from build123d import *

# Parameters (mm, degrees)
F0_W     = 550
F0_H     = 400
F1_DEPTH = 10
F2_W     = 9
F2_H     = 20
F2_H_2   = 70
F2_H_3   = 10
F2_H_4   = 75
F2_H_5   = 15
F2_H_6   = 18
F3_DEPTH = 5


with BuildPart() as f1:
    # F0 (on Front) → F1 (new body)
    with BuildSketch(Plane.XZ):
        Rectangle(F0_W, F0_H)
    extrude(amount=F1_DEPTH)

    # F2 (on face) → F3 (cut)
    with BuildSketch(Plane.XZ.offset(10)):
        Polygon((-218.013464, -37.5), (-215.013464, -37.5), (-215.013464, 37.5), (-218.013464, 37.5), (-227.013464, 37.5), (-230.013464, 37.5), (-230.013464, -37.5), (-227.013464, -37.5), align=None)
        with Locations((-222.513464, -47.5)):
            Rectangle(F2_W, F2_H)
        with Locations((-222.513464, 72.5)):
            Rectangle(F2_W, F2_H_2)
        Polygon((219.224181, -40.562903), (222.224181, -40.562903), (222.224181, 29.437097), (219.224181, 29.437097), (210.224181, 29.437097), (207.224181, 29.437097), (207.224181, -40.562903), (210.224181, -40.562903), align=None)
        with Locations((214.724181, -45.562903)):
            Rectangle(F2_W, F2_H_3)
        with Locations((214.724181, 66.937097)):
            Rectangle(F2_W, F2_H_4)
        Polygon((-172.425557, -35.359889), (-169.425557, -35.359889), (-169.425557, 29.640111), (-172.425557, 29.640111), (-181.425557, 29.640111), (-184.425557, 29.640111), (-184.425557, -35.359889), (-181.425557, -35.359889), align=None)
        with Locations((-176.925557, -40.359889)):
            Rectangle(F2_W, F2_H_3)
        with Locations((-176.925557, 67.140111)):
            Rectangle(F2_W, F2_H_4)
        Polygon((-124.808628, -20.359889), (-121.808628, -20.359889), (-121.808628, 59.640111), (-124.808628, 59.640111), (-133.808628, 59.640111), (-136.808628, 59.640111), (-136.808628, -20.359889), (-133.808628, -20.359889), align=None)
        with Locations((-129.308628, -27.859889)):
            Rectangle(F2_W, F2_H_5)
        with Locations((-129.308628, 69.640111)):
            Rectangle(F2_W, F2_H)
        Polygon((-73.533672, -28.500006), (-70.533672, -28.500006), (-70.533672, 36.499994), (-73.533672, 36.499994), (-82.533672, 36.499994), (-85.533672, 36.499994), (-85.533672, -28.500006), (-82.533672, -28.500006), align=None)
        with Locations((-78.033672, -33.500006)):
            Rectangle(F2_W, F2_H_3)
        with Locations((-78.033672, 41.499994)):
            Rectangle(F2_W, F2_H_3)
        Polygon((-19.896116, -21.071613), (-16.896116, -21.071613), (-16.896116, 38.928387), (-19.896116, 38.928387), (-28.896116, 38.928387), (-31.896116, 38.928387), (-31.896116, -21.071613), (-28.896116, -21.071613), align=None)
        with Locations((-24.396116, -28.571613)):
            Rectangle(F2_W, F2_H_5)
        with Locations((-24.396116, 43.928387)):
            Rectangle(F2_W, F2_H_3)
        Polygon((46.493838, -21.071613), (49.493838, -21.071613), (49.493838, 38.928387), (46.493838, 38.928387), (37.493838, 38.928387), (34.493838, 38.928387), (34.493838, -21.071613), (37.493838, -21.071613), align=None)
        with Locations((41.993838, -28.571613)):
            Rectangle(F2_W, F2_H_5)
        with Locations((41.993838, 43.928387)):
            Rectangle(F2_W, F2_H_3)
        Polygon((108.827169, -24.357102), (111.827169, -24.357102), (111.827169, 35.642898), (108.827169, 35.642898), (99.827169, 35.642898), (96.827169, 35.642898), (96.827169, -24.357102), (99.827169, -24.357102), align=None)
        with Locations((104.327169, -29.357102)):
            Rectangle(F2_W, F2_H_3)
        with Locations((104.327169, 44.642898)):
            Rectangle(F2_W, F2_H_6)
        Polygon((164.842565, -29.71177), (167.842565, -29.71177), (167.842565, 40.28823), (164.842565, 40.28823), (155.842565, 40.28823), (152.842565, 40.28823), (152.842565, -29.71177), (155.842565, -29.71177), align=None)
        with Locations((160.342565, -34.71177)):
            Rectangle(F2_W, F2_H_3)
        with Locations((160.342565, 47.78823)):
            Rectangle(F2_W, F2_H_5)
    extrude(amount=-F3_DEPTH, mode=Mode.SUBTRACT)


solid = f1.part
The model under review builds one solid part; all positions refer to its coordinate system, in mm. Coordinates: 2 decimals unless noted, no trailing zeros. Loops run counter-clockwise (first coordinate to the right, second up) from the corner with the lowest first, then second, coordinate; pieces in that order, holes last. Notation, with made-up numbers: (74, 46.25) -> (109, 46.25) arc R23 cw to (109, 65.25) -> close; hole circle Ø4 at (1.5, -10). An arc over 180 degrees is marked (long way). Use a Markdown table: item, result. Add a question column.
1. Draft analysis for pull direction X (two halves, no side actions). For faces 1 (the face through (-4, 0, 3)), 2 (the face through (42, -5, 7)), state which applies: pulls with the +X half, pulls with the -X half, needs draft (parallel to the pull), parting line crosses it, or undercut.
2. To check wall thickness, follow line 1 (X direction, y = -7, z = -43.5); line 2 (Z direction, x = -129, y = -7.75); line 3 (Y direction, x = -126, z = 43). State the ranges of each line that lie inside material, in increasing order.
3. Add section A-A on z = 86.5. Write out the cut boundary in (x, y).
4. Add section B-B on y = -8.5. Give the number of separate pieces and of enclosed holes in the cut face, plus the area to 3 significant figures.
5. Clearance check with a flat-ended pin moving along its axis: pin 1 Ø4.5 at (x, z) = (-176.5, 56) entering from -Y. State where the tip first meets the part, or that it passes through.
Returned:
| question | item | result |
|---|---|---|
| 1 | face 1 | needs draft |
| 1 | face 2 | undercut |
| 2 | line 1 | x = -275 to -227.01, -218.01 to -181.43, -172.43 to 210.22, 219.22 to 275 |
| 2 | line 2 | z = -200 to -35.36, 79.64 to 200 |
| 2 | line 3 | y = -5 to 0 |
| 3 | outline | (-275, -10) -> (-227.01, -10) -> (-227.01, -5) -> (-218.01, -5) -> (-218.01, -10) -> (-181.43, -10) -> (-181.43, -5) -> (-172.43, -5) -> (-172.43, -10) -> (210.22, -10) -> (210.22, -5) -> (219.22, -5) -> (219.22, -10) -> (275, -10) -> (275, 0) -> (-275, 0) -> close |
| 4 | separate pieces | 1 |
| 4 | enclosed holes | 9 |
| 4 | area | 207,000 mm² |
| 5 | pin 1 | stops at y = -5 |
